Geometry check sheet. Reference: the model listing, model coordinates, mm. A direction names the side the tool comes from. Give positions to 0.01 mm unless a question says otherwise; leave off trailing zeros. Loops run counter-clockwise (first coordinate to the right, second up) from the corner with the lowest first, then second, coordinate; pieces in that order, holes last. Notation, with made-up numbers: (-19.5, 63) - (-15.5, 63) arc R14 ccw to (-15.5, 87) - close; hole circle Ø6 at (16.5, 37.5). An arc over 180 degrees is marked (long way). Use a Markdown table: item, result. Add a question column.
1. Draft check along Z on faces 1 (the flat face through (-1, 2, -100)), 2 (the flat face through (52, 2, -24.412)), 3 (the flat face through (1, 0, -1)). Enter one of: pulls with the +Z half, pulls with the -Z half, needs draft (parallel to the pull), parting line crosses it, or undercut.
2. Set-up check for faces 4 (the flat face through (-75, 2, 1)), 5 (the flat face through (22, 2, -64.588)): record each of +Z, -Z, +X, -X, +Y, -Y from which the full face is reachable in a straight line by a thin tool's end or side.
3. Cross-section at B-B on y = 0.7. Count the separate pieces of the cut face and the enclosed holes in it, and give its area (3 significant figures).
4. Cross-section at A-A on x = 54.5. Enter the section's corners in (y, z), and give its area (3 significant figures).
5. Material ranges on L1, parallel to Z at x = 69, y = 1; L2, parallel to X at y = 1.8, z = -94; L3, parallel to Z at x = 46.5, y = 2.3, recorded low to high.
6. Depth check by flat-ended pin: P1, Ø3.5, axis at x = -69, z = 34, coming from the +Y side. Enter the tip coordinate at first touch or a pass-through.
from build123d import *

# Parameters (mm, degrees)
EXTRUDE_1_DEPTH     = 4
SKETCH_3_R          = 1.5875
CUT_EXTRUDE_2_DEPTH = 126.063983624
CUT_EXTRUDE_3_DEPTH = 126.063983624


with BuildPart() as part:
    # Эскиз1 → Бобышка-Вытянуть1 (new body)
    with BuildSketch(Plane(origin=(0, 0, 0), x_dir=(1, 0, 0), z_dir=(0, 1, 0))):
        with BuildLine():
            Line((-72, 100), (72, 100))
            ThreePointArc((72, 100), (74.121320344, 99.121320344), (75, 97))
            Line((75, 97), (75, -97))
            ThreePointArc((75, -97), (74.121320344, -99.121320344), (72, -100))
            Line((72, -100), (-72, -100))
            ThreePointArc((-72, -100), (-74.121320344, -99.121320344), (-75, -97))
            Line((-75, -97), (-75, 97))
            ThreePointArc((-75, 97), (-74.121320344, 99.121320344), (-72, 100))
        make_face()
    extrude(amount=EXTRUDE_1_DEPTH)

    # Эскиз3 → Вырез-Вытянуть2 (cut, through all)
    with BuildSketch(Plane(origin=(0, 4, 0), x_dir=(1, 0, 0), z_dir=(0, 1, 0))):
        with Locations(Location((-69, 94, 0), (0, 0, 270))):
            Circle(SKETCH_3_R)
        with Locations(Location((0, 94, 0), (0, 0, 270))):
            Circle(SKETCH_3_R)
        with Locations(Location((69, 94, 0), (0, 0, 270))):
            Circle(SKETCH_3_R)
        with Locations(Location((-69, -34, 0), (0, 0, 90))):
            Circle(SKETCH_3_R)
        with Locations(Location((69, -34, 0), (0, 0, 90))):
            Circle(SKETCH_3_R)
        with Locations(Location((0, -34, 0), (0, 0, 90))):
            Circle(SKETCH_3_R)
        with Locations(Location((69, -94, 0), (0, 0, 90))):
            Circle(SKETCH_3_R)
        with Locations(Location((0, -94, 0), (0, 0, 90))):
            Circle(SKETCH_3_R)
        with Locations(Location((-69, -94, 0), (0, 0, 90))):
            Circle(SKETCH_3_R)
        with Locations(Location((0, 34, 0), (0, 0, 270))):
            Circle(SKETCH_3_R)
        with Locations(Location((69, 34, 0), (0, 0, 270))):
            Circle(SKETCH_3_R)
        with Locations(Location((-69, 34, 0), (0, 0, 270))):
            Circle(SKETCH_3_R)
    extrude(amount=-CUT_EXTRUDE_2_DEPTH, mode=Mode.SUBTRACT)

    # Эскиз2 → Вырез-Вытянуть3 (cut, through all)
    with BuildSketch(Plane(origin=(0, 4, 0), x_dir=(1, 0, 0), z_dir=(0, 1, 0))):
        with BuildLine():
            Line((-32, 64.5875), (-12, 64.5875))
            ThreePointArc((-12, 64.5875), (-10.4125, 63), (-12, 61.4125))
            Line((-12, 61.4125), (-32, 61.4125))
            ThreePointArc((-32, 61.4125), (-33.5875, 63), (-32, 64.5875))
        make_face()
        with BuildLine():
            Line((-58, 64.5875), (-38, 64.5875))
            ThreePointArc((-38, 64.5875), (-36.4125, 63), (-38, 61.4125))
            Line((-38, 61.4125), (-58, 61.4125))
            ThreePointArc((-58, 61.4125), (-59.5875, 63), (-58, 64.5875))
        make_face()
        with BuildLine():
            Line((-28, 27.5875), (-8, 27.5875))
            ThreePointArc((-8, 27.5875), (-6.4125, 26), (-8, 24.4125))
            Line((-8, 24.4125), (-28, 24.4125))
            ThreePointArc((-28, 24.4125), (-29.5875, 26), (-28, 27.5875))
        make_face()
        with BuildLine():
            Line((-62, 27.5875), (-42, 27.5875))
            ThreePointArc((-42, 27.5875), (-40.4125, 26), (-42, 24.4125))
            Line((-42, 24.4125), (-62, 24.4125))
            ThreePointArc((-62, 24.4125), (-63.5875, 26), (-62, 27.5875))
        make_face()
        with BuildLine():
            Line((62, 24.4125), (42, 24.4125))
            ThreePointArc((42, 24.4125), (40.4125, 26), (42, 27.5875))
            Line((42, 27.5875), (62, 27.5875))
            ThreePointArc((62, 27.5875), (63.5875, 26), (62, 24.4125))
        make_face()
        with BuildLine():
            Line((28, 24.4125), (8, 24.4125))
            ThreePointArc((8, 24.4125), (6.4125, 26), (8, 27.5875))
            Line((8, 27.5875), (28, 27.5875))
            ThreePointArc((28, 27.5875), (29.5875, 26), (28, 24.4125))
        make_face()
        with BuildLine():
            Line((58, 61.4125), (38, 61.4125))
            ThreePointArc((38, 61.4125), (36.4125, 63), (38, 64.5875))
            Line((38, 64.5875), (58, 64.5875))
            ThreePointArc((58, 64.5875), (59.5875, 63), (58, 61.4125))
        make_face()
        with BuildLine():
            Line((32, 61.4125), (12, 61.4125))
            ThreePointArc((12, 61.4125), (10.4125, 63), (12, 64.5875))
            Line((12, 64.5875), (32, 64.5875))
            ThreePointArc((32, 64.5875), (33.5875, 63), (32, 61.4125))
        make_face()
    extrude(amount=-CUT_EXTRUDE_3_DEPTH, mode=Mode.SUBTRACT)


solid = part.part
Values found:
| question | item | result |
|---|---|---|
| 1 | face 1 | pulls with the -Z half |
| 1 | face 2 | undercut |
| 1 | face 3 | needs draft |
| 2 | face 4 | +Z, -Z, -X, +Y, -Y |
| 2 | face 5 | +Y, -Y |
| 3 | separate pieces | 1 |
| 3 | enclosed holes | 20 |
| 3 | area | 29,300 mm2 |
| 4 | outline | (0, -100) - (4, -100) - (4, -64.59) - (0, -64.59) - close; (0, -61.41) - (4, -61.41) - (4, -27.59) - (0, -27.59) - close; (0, -24.41) - (4, -24.41) - (4, 100) - (0, 100) - close |
| 4 | area | 775 mm2 |
| 5 | L1 | z = -100 to -95.59, -92.41 to -35.59, -32.41 to 32.41, 35.59 to 92.41, 95.59 to 100 |
| 5 | L2 | x = -75 to -70.59, -67.41 to -1.59, 1.59 to 67.41, 70.59 to 75 |
| 5 | L3 | z = -100 to -64.59, -61.41 to -27.59, -24.41 to 100 |
| 6 | P1 | stops at y = 4 |
